Here's how the part is built. I have some questions about the finished solid (model axes, mm). A direction names the side the tool comes from. Round coordinates to 2 decimals unless told otherwise and drop trailing zeros. Order: outer loops, then holes, each group sorted by start corner. A loop starts at its lowest first (then second) coordinate and runs counter-clockwise, first axis right, second up.
```python
from build123d import *

# Parameters (mm, degrees)
F1_DEPTH = 25
F2_DEPTH = 10
F3_R     = 5
F5_DEPTH = 3


with BuildPart() as f1:
    # F0 (on Front) → F1 (new body)
    with BuildSketch(Plane.XZ):
        with BuildLine():
            ThreePointArc((17.496143, -0.367408), (16.137561, 2.845487), (16.315335, 6.329284))
            ThreePointArc((16.315335, 6.329284), (15.155445, 8.75), (13.638989, 10.964853))
            ThreePointArc((13.638989, 10.964853), (10.533045, 12.552794), (8.429886, 15.335808))
            ThreePointArc((8.429886, 15.335808), (5.985353, 16.444621), (3.4, 17.166537))
            ThreePointArc((3.4, 17.166537), (0, 16.386509), (-3.4, 17.166537))
            ThreePointArc((-3.4, 17.166537), (-5.985353, 16.444621), (-8.429886, 15.335808))
            ThreePointArc((-8.429886, 15.335808), (-10.533045, 12.552794), (-13.638989, 10.964853))
            ThreePointArc((-13.638989, 10.964853), (-15.155445, 8.75), (-16.315335, 6.329284))
            ThreePointArc((-16.315335, 6.329284), (-16.137561, 2.845487), (-17.496143, -0.367408))
            ThreePointArc((-17.496143, -0.367408), (-17.234136, -3.038843), (-16.566657, -5.638782))
            ThreePointArc((-16.566657, -5.638782), (-14.191133, -8.193254), (-13.166657, -11.527755))
            ThreePointArc((-13.166657, -11.527755), (-11.248783, -13.405778), (-9.066256, -14.9684))
            ThreePointArc((-9.066256, -14.9684), (-5.604516, -15.398281), (-2.676347, -17.294137))
            ThreePointArc((-2.676347, -17.294137), (0, -17.5), (2.676347, -17.294137))
            ThreePointArc((2.676347, -17.294137), (5.604516, -15.398281), (9.066256, -14.9684))
            ThreePointArc((9.066256, -14.9684), (11.248783, -13.405778), (13.166657, -11.527755))
            ThreePointArc((13.166657, -11.527755), (14.191133, -8.193254), (16.566657, -5.638782))
            ThreePointArc((16.566657, -5.638782), (17.234136, -3.038843), (17.496143, -0.367408))
        make_face()
        with BuildLine():
            ThreePointArc((4, 3), (4.743416, 1.581139), (5, 0))
            ThreePointArc((5, 0), (-1.581139, -4.743416), (-4, 3))
            ThreePointArc((-4, 3), (0, 5), (4, 3))
        make_face(mode=Mode.SUBTRACT)
        with BuildLine():
            ThreePointArc((-4, 3), (-1.581139, -4.743416), (5, 0))
            ThreePointArc((5, 0), (4.743416, 1.581139), (4, 3))
            Line((4, 3), (-4, 3))
        make_face()
        with BuildLine():
            Line((-4, 3), (4, 3))
            ThreePointArc((4, 3), (0, 5), (-4, 3))
        make_face()
    extrude(amount=F1_DEPTH)

    # F0 (on Front) → F2 (cut)
    with BuildSketch(Plane.XZ):
        with BuildLine():
            ThreePointArc((-4, 3), (-1.581139, -4.743416), (5, 0))
            ThreePointArc((5, 0), (4.743416, 1.581139), (4, 3))
            Line((4, 3), (-4, 3))
        make_face()
    extrude(amount=F2_DEPTH, mode=Mode.SUBTRACT)

    # F3
    f3_edges = [f1.edges().sort_by_distance(p)[0] for p in [
        (16.137561, -25, 2.845487),
        (15.155445, -25, 8.75),
        (10.533045, -25, 12.552794),
        (5.985353, -25, 16.444621),
        (0, -25, 16.386509),
        (-5.985353, -25, 16.444621),
        (-10.533045, -25, 12.552794),
        (-15.155445, -25, 8.75),
        (-16.137561, -25, 2.845487),
        (-17.234136, -25, -3.038843),
        (-14.191133, -25, -8.193254),
        (-11.248783, -25, -13.405778),
        (-5.604516, -25, -15.398281),
        (0, -25, -17.5),
        (5.604516, -25, -15.398281),
        (11.248783, -25, -13.405778),
        (14.191133, -25, -8.193254),
        (17.234136, -25, -3.038843),
    ]]
    fillet(f3_edges, radius=F3_R)

    # F4 (on face) → F5 (cut)
    with BuildSketch(Plane.XZ.offset(25)):
        Polygon((-3.125, 0), (0, 0), (3.125, 0), (0, 9.25), align=None)
    extrude(amount=-F5_DEPTH, mode=Mode.SUBTRACT)


solid = f1.part
```
1. I'm going to push flat-ended pins straight in: P1, Ø2, axis at y = -15, z = -5, coming from the +X side; P2, Ø1, axis at x = 5.5, y = -5.5, coming from the +Z side; P3, Ø2.5, axis at x = -0.5, z = -0.5, coming from the +Y side. Where does each tip first touch, or does it pass through?
Evaluation:
P1: stops at x = 17.04
P2: stops at z = 16.77
P3: stops at y = -10
2. If we section it at A-A, the plane y = -7.75: Write out the boundary of the cut face in (x, z).
Evaluation:
outline: (-17.5, -0.37) arc R17.5 ccw to (-16.57, -5.64) arc R7.8 cw to (-13.17, -11.53) arc R17.5 ccw to (-9.07, -14.97) arc R7.8 cw to (-2.68, -17.29) arc R17.5 ccw to (2.68, -17.29) arc R7.8 cw to (9.07, -14.97) arc R17.5 ccw to (13.17, -11.53) arc R7.8 cw to (16.57, -5.64) arc R17.5 ccw to (17.5, -0.37) arc R7.8 cw to (16.32, 6.33) arc R17.5 ccw to (13.64, 10.96) arc R7.8 cw to (8.43, 15.34) arc R17.5 ccw to (3.4, 17.17) arc R7.8 cw to (-3.4, 17.17) arc R17.5 ccw to (-8.43, 15.34) arc R7.8 cw to (-13.64, 10.96) arc R17.5 ccw to (-16.32, 6.33) arc R7.8 cw to start; hole (-4, 3) arc R5 ccw (long way) to (5, 0) arc R5 ccw to (4, 3) - close
3. I need wall thicknesses on probe 1 along Z at (x, y) = (0, -5.25); probe 2 along Y at (x, z) = (1, -12.5); probe 3 along Y at (x, z) = (-4.5, 0). Which ranges of each line are inside material? Lowest first, please.
Evaluation:
probe 1: z = -17.5 to -5, 3 to 16.39
probe 2: y = -24.99 to 0
probe 3: y = -25 to -10
4. On a 3-axis mill with a long thin cutter (end or side, diameter ignored), from which of +Z, -Z, +X, -X, +Y, -Y can I reach the whole of each face in a straight line? I mean faces 1 (the cylindrical face through (16.146, -9.86, 2.797)), 2 (the flat face through (0, -10, -1)), 3 (the flat face through (1.584, -23.521, 4.56)). Say none if no direction works.
Evaluation:
face 1: +X, +Y, -Y
face 2: +Y
face 3: -Y
5. If we section it at B-B, the plane y = -19.5: Write out the boundary of the cut face in (x, z), and give its area (3 significant figures).
Evaluation:
outline: (-17.5, -0.37) arc R17.5 ccw to (-16.57, -5.64) arc R7.8 cw to (-13.17, -11.53) arc R17.5 ccw to (-9.07, -14.97) arc R7.8 cw to (-2.68, -17.29) arc R17.5 ccw to (2.68, -17.29) arc R7.8 cw to (9.07, -14.97) arc R17.5 ccw to (13.17, -11.53) arc R7.8 cw to (16.57, -5.64) arc R17.5 ccw to (17.5, -0.37) arc R7.8 cw to (16.32, 6.33) arc R17.5 ccw to (13.64, 10.96) arc R7.8 cw to (8.43, 15.34) arc R17.5 ccw to (3.4, 17.17) arc R7.8 cw to (-3.4, 17.17) arc R17.5 ccw to (-8.43, 15.34) arc R7.8 cw to (-13.64, 10.96) arc R17.5 ccw to (-16.32, 6.33) arc R7.8 cw to start
area: 916 mm2
6. If we mould it in two halves opening along Z, with no side actions, what happens to faces 4 (the flat face through (0, -5, 3)), 5 (the cylindrical face through (17.228, -9.86, -3.076)), 6 (the flat face through (0, -25, -3))? For each: released by +Z, released by -Z, zero draft, split by the parting line, or undercut.
Evaluation:
face 4: undercut
face 5: released by -Z
face 6: zero draft
